from build123d import *

# Parameters (mm, degrees)
EXTRUDE_THIN1_DEPTH = 30
CUT_EXTRUDE1_DEPTH  = 1
LPATTERN1_COUNT     = 2
LPATTERN1_PITCH     = 25


with BuildPart() as part:
    # Sketch1 → Extrude-Thin1 (new body)
    with BuildSketch(Plane(origin=(0, 0, 0), x_dir=(0, 0, -1), z_dir=(1, 0, 0))):
        with BuildLine():
            Line((-17.5, 6.5), (-15.5, 6.5))
            ThreePointArc((-15.5, 6.5), (-14.085786438, 5.914213562), (-13.5, 4.5))
            Line((-13.5, 4.5), (-13.5, 2))
            ThreePointArc((-13.5, 2), (-12.914213562, 0.585786438), (-11.5, 0))
            Line((-11.5, 0), (11.5, 0))
            ThreePointArc((11.5, 0), (12.914213562, 0.585786438), (13.5, 2))
            Line((13.5, 2), (13.5, 4.5))
            ThreePointArc((13.5, 4.5), (14.085786438, 5.914213562), (15.5, 6.5))
            Line((15.5, 6.5), (17.5, 6.5))
            Line((17.5, 6.5), (17.5, 7.5))
            Line((17.5, 7.5), (15.5, 7.5))
            ThreePointArc((15.5, 7.5), (13.378679656, 6.621320344), (12.5, 4.5))
            Line((12.5, 4.5), (12.5, 2))
            ThreePointArc((12.5, 2), (12.207106781, 1.292893219), (11.5, 1))
            Line((11.5, 1), (-11.5, 1))
            ThreePointArc((-11.5, 1), (-12.207106781, 1.292893219), (-12.5, 2))
            Line((-12.5, 2), (-12.5, 4.5))
            ThreePointArc((-12.5, 4.5), (-13.378679656, 6.621320344), (-15.5, 7.5))
            Line((-15.5, 7.5), (-17.5, 7.5))
            Line((-17.5, 7.5), (-17.5, 6.5))
        make_face()
    extrude(amount=EXTRUDE_THIN1_DEPTH)

    # Sketch2 → Cut-Extrude1 (cut)
    with BuildSketch(Plane.XZ):
        with BuildLine():
            Line((-5.875, 3.125), (5.875, 3.125))
            ThreePointArc((5.875, 3.125), (9, 0), (5.875, -3.125))
            Line((5.875, -3.125), (-5.875, -3.125))
            ThreePointArc((-5.875, -3.125), (-9, 0), (-5.875, 3.125))
        make_face()
    cut_extrude1 = extrude(amount=-CUT_EXTRUDE1_DEPTH, mode=Mode.SUBTRACT)

    # LPattern1: Cut-Extrude1 ×2
    with Locations(*[(i * LPATTERN1_PITCH, 0, 0) for i in range(1, LPATTERN1_COUNT)]):
        add(cut_extrude1, mode=Mode.SUBTRACT)


solid = part.part
Build history of the part. All positions in model axes, mm. A direction names the side the tool comes from. Give positions to 0.01 mm unless a question says otherwise; leave off trailing zeros. Loops run counter-clockwise (first coordinate to the right, second up) from the corner with the lowest first, then second, coordinate; pieces in that order, holes last. Notation, with made-up numbers: (87, 41) -> (91, 41) arc R16 cw to (91, 52) -> close; hole circle Ø2 at (87.5, -16.75). An arc over 180 degrees is marked (long way). Answer in a Markdown table with one row per item.
Item 1: Tool access for faces 4 (the flat face through (15, 3, 13.5)), 5 (the flat face through (15, 7, -17.5)), 6 (the flat face through (2.9, 0.5, 3.125)), 7 (the flat face through (15, 3, -12.5)), 8 (the flat face through (24.6, 0.5, -3.125)): list every direction of +Z, -Z, +X, -X, +Y, -Y with a clear straight run to the whole face (end or side of a thin tool).
Findings below:
| item | result |
|---|---|
| face 4 | +Z, +X, -X, -Y |
| face 5 | -Z, +X, -X, +Y, -Y |
| face 6 | -X, +Y, -Y |
| face 7 | +X, -X, +Y |
| face 8 | +X, +Y, -Y |
Item 2: Slice it at B-B on y = 3. Write the cut outline in (x, z), plus the area to 3 significant figures.
Findings below:
| item | result |
|---|---|
| outline | (0, -13.5) -> (30, -13.5) -> (30, -12.5) -> (0, -12.5) -> close; (0, 12.5) -> (30, 12.5) -> (30, 13.5) -> (0, 13.5) -> close |
| area | 60.0 mm² |
Item 3: Slice it at D-D on y = 0.5. Write the cut outline in (x, z) (3 decimals), plus the area to 3 significant figures.
Findings below:
| item | result |
|---|---|
| outline | (0, -12.823) -> (30, -12.823) -> (30, -3.125) -> (19.125, -3.125) arc R3.125 cw to (19.125, 3.125) -> (30, 3.125) -> (30, 12.823) -> (0, 12.823) -> (0, 3.125) -> (5.875, 3.125) arc R3.125 cw to (5.875, -3.125) -> (0, -3.125) -> close |
| area | 634 mm² |
Item 4: Slice it at C-C on x = 12.5. Write the cut outline in (y, z).
Findings below:
| item | result |
|---|---|
| outline | (0, -11.5) arc R2 ccw to (2, -13.5) -> (4.5, -13.5) arc R2 cw to (6.5, -15.5) -> (6.5, -17.5) -> (7.5, -17.5) -> (7.5, -15.5) arc R3 ccw to (4.5, -12.5) -> (2, -12.5) arc R1 cw to (1, -11.5) -> (1, 11.5) arc R1 cw to (2, 12.5) -> (4.5, 12.5) arc R3 ccw to (7.5, 15.5) -> (7.5, 17.5) -> (6.5, 17.5) -> (6.5, 15.5) arc R2 cw to (4.5, 13.5) -> (2, 13.5) arc R2 ccw to (0, 11.5) -> close |
Item 5: Slice it at A-A on x = 20. Write the cut outline in (y, z) (3 decimals), plus the area to 3 significant figures.
Findings below:
| item | result |
|---|---|
| outline | (0, -11.5) arc R2 ccw to (2, -13.5) -> (4.5, -13.5) arc R2 cw to (6.5, -15.5) -> (6.5, -17.5) -> (7.5, -17.5) -> (7.5, -15.5) arc R3 ccw to (4.5, -12.5) -> (2, -12.5) arc R1 cw to (1, -11.5) -> (1, -3.125) -> (0, -3.125) -> close; (0, 3.125) -> (1, 3.125) -> (1, 11.5) arc R1 cw to (2, 12.5) -> (4.5, 12.5) arc R3 ccw to (7.5, 15.5) -> (7.5, 17.5) -> (6.5, 17.5) -> (6.5, 15.5) arc R2 cw to (4.5, 13.5) -> (2, 13.5) arc R2 ccw to (0, 11.5) -> close |
| area | 38.3 mm² |
Item 6: Probe line 1 along Z through (x, y) = (17.75, 3.25); line 2 along Y through (x, z) = (19.75, -10); line 3 along Z through (x, y) = (25, 5). List the from-to ranges inside material, lowest first. Write a range as [from, to].
Findings below:
| item | result |
|---|---|
| line 1 | z = [-13.5, -12.5], [12.5, 13.5] |
| line 2 | y = [0, 1] |
| line 3 | z = [-13.56, -12.54], [12.54, 13.56] |
Item 7: Flat gauge pins, fed straight in: P1, Ø0.6, axis at x = 19.5, z = -16.5, coming from the -Y side; P2, Ø12, axis at x = 11, z = -2, coming from the +Y side; P3, Ø2, axis at x = 19.5, y = 2.5, coming from the +Z side; P4, Ø6, axis at x = 26, z = -8.5, coming from the -Y side. Where does each tip first touch, or does it go through?
Findings below:
| item | result |
|---|---|
| P1 | stops at y = 6.5 |
| P2 | stops at y = 1 |
| P3 | stops at z = 13.5 |
| P4 | stops at y = 0 |
Item 8: Mould opens along Z. For faces 1 (the flat face through (15, 3, 12.5)), 2 (the flat face through (15, 7, 17.5)), 3 (the flat face through (15, 6.5, 17)) say: pulls with the +Z half, pulls with the -Z half, needs draft (parallel to the pull), parting line crosses it, or undercut.
Findings below:
| item | result |
|---|---|
| face 1 | undercut |
| face 2 | pulls with the +Z half |
| face 3 | needs draft |
